Autodesk Inventor part; units mm, degrees
ref_plane "YZ Plane" through (0, 0, 0) normal (1, 0, 0) x (0, 1, 0)
ref_plane "XZ Plane" through (0, 0, 0) normal (0, 1, 0) x (-1, 0, 0)
ref_plane "XY Plane" through (0, 0, 0) normal (0, 0, 1) x (1, 0, 0)
sketch "Boceto1" plane through (0, 0, 0) normal (0, 1, 0) x (-1, 0, 0)
  line L0 (-71.0974, 28.13) -> (-71.0974, -25.87)
  line L1 (-71.0974, -25.87) -> (27.9026, -25.87)
  line L2 (27.9026, -25.87) -> (27.9026, 28.13)
  line L3 (4.4026, 48.13) -> (-47.5974, 48.13)
  line L4 (-47.5974, 48.13) -> (-47.5974, 28.13)
  line L5 (4.4026, 28.13) -> (4.4026, 48.13)
  line L6 (27.9026, 28.13) -> (4.4026, 28.13)
  line L7 (-47.5974, 28.13) -> (-71.0974, 28.13)
  circle A0 centre (-5.5974, 32.13) radius 2
  line L8 (-21.5974, 48.13) -> (-21.5974, -25.87)
  circle A1 centre (-37.5974, 32.13) radius 2
  line L9 (22.9026, -12.37) -> (6.9026, -12.37)
  line L10 (6.9026, -12.37) -> (6.9026, -23.37)
  line L11 (6.9026, -23.37) -> (22.9026, -23.37)
  line L12 (22.9026, -23.37) -> (22.9026, -12.37)
  line L13 (-66.0974, -12.37) -> (-50.0974, -12.37)
  line L14 (-50.0974, -12.37) -> (-50.0974, -23.37)
  line L15 (-50.0974, -23.37) -> (-66.0974, -23.37)
  line L16 (-66.0974, -23.37) -> (-66.0974, -12.37)
  circle A2 centre (-8.0974, -16.37) radius 2
  circle A3 centre (-35.0974, -16.37) radius 2
  point P0 (0, 0)
  dimension "d0" = 54
  dimension "d1" = 99
  dimension "d2" = 20
  dimension "d3" = 52
  dimension "d4" = 23.5
  dimension "d5" = 23.5
  dimension "d6" = 4
  dimension "d7" = 16
  dimension "d8" = 10
  dimension "d9" = 2.5
  dimension "d10" = 5
  dimension "d11" = 11
  dimension "d12" = 16
  dimension "d13" = 4
  dimension "d15" = 9.5
  dimension "d18" = 34
  dimension "d19" = 15
extrude "Extrusión1" add sketch "Boceto1" along normal blind 3.4
equation "\"Radio_pliegue\" = Grosor"
equation "\"Anchura_desahogo_plegado\" = Grosor"
equation "\"Profundidad_desahogo_plegado\" = 0.5 * Grosor"
equation "\"Tamaño_destalonado\" = 4 * Grosor"
equation "\"Remanente_mínimo\" = 2 * Grosor"
equation "\"Radiodetransición\" = Radio_pliegue"
equation "\"Tamaño_de_radio_de_Jacobi\" = Radio_pliegue"
equation "\"TamañoSeparación\" = Grosor"
properties part number "PlacaInferior"
Work out the finished part from the listing and answer in its coordinate system (mm). A direction names the side the tool comes from. Give positions to 0.01 mm unless a question says otherwise; leave off trailing zeros. Loops run counter-clockwise (first coordinate to the right, second up) from the corner with the lowest first, then second, coordinate; pieces in that order, holes last. Notation, with made-up numbers: (17, 32) - (61, 32) arc R11 ccw to (61, 38) - close; hole circle Ø5 at (82, 14). An arc over 180 degrees is marked (long way). Answer in a Markdown table with one row per item. Add a question column.
Q1. A tool of negligible diameter and unlimited length cuts with its end or side. For faces 5 (the flat face through (59, 2, 28.13)), 6 (the flat face through (-16, 2, 28.13)), 7 (the flat face through (22, 2, -25.87)), 8 (the flat face through (-27.903, 2, 1)), 9 (the flat face through (58, 2, -12.37)), from which of +Z, -Z, +X, -X, +Y, -Y can it reach the whole face along a straight path? Write none if from no direction.
Q2. Determine the mould class of faces 1 (the cylindrical face through (37.095, 1.676, -16.458)), 2 (the flat face through (58, 2, -23.37)), 3 (the flat face through (47.597, 2, 38)), 4 (the flat face through (22, 3.4, 12)) for opening direction X: released by +X, released by -X, zero draft, split by the parting line, or undercut.
Q3. The part is cut by section A-A (z = -16.37). Determine the outline of the cut face in (x, y).
Q4. The part is cut by section C-C (z = 32.13). Determine the outline of the cut face in (x, y), and give its area (3 significant figures).
Q5. Each of these flat-tipped pins is pushed along its axis until it touches: P1, Ø1.7, axis at x = 63, y = 2, coming from the +Z side; P2, Ø1, axis at y = 2.5, z = 38.5, coming from the +X side; P3, Ø6, axis at x = 14, z = 36, coming from the -Y side. Where does it stop, or does it pass through?
Q6. The part is cut by section B-B (y = 2.8). Determine the outline of the cut face in (x, z), and give its area (3 significant figures).
Q7. Consider line 1 along X through (y, z) = (1.5, -19); line 2 along Z through (x, y) = (-13, 1.5); line 3 along X through (y, z) = (1.85, 30.5). Determine where each line is inside the solid, lowest interval first.
Q8. The part is cut by section D-D (z = 43.5). Determine the outline of the cut face in (x, y), and give its area (3 significant figures).
Solution:
| question | item | result |
|---|---|---|
| 1 | face 5 | +Z, +X, +Y, -Y |
| 1 | face 6 | +Z, -X, +Y, -Y |
| 1 | face 7 | -Z, +X, -X, +Y, -Y |
| 1 | face 8 | +Z, -Z, -X, +Y, -Y |
| 1 | face 9 | +Y, -Y |
| 2 | face 1 | undercut |
| 2 | face 2 | undercut |
| 2 | face 3 | released by +X |
| 2 | face 4 | zero draft |
| 3 | outline | (-27.9, 0) - (-22.9, 0) - (-22.9, 3.4) - (-27.9, 3.4) - close; (-6.9, 0) - (6.1, 0) - (6.1, 3.4) - (-6.9, 3.4) - close; (10.1, 0) - (33.1, 0) - (33.1, 3.4) - (10.1, 3.4) - close; (37.1, 0) - (50.1, 0) - (50.1, 3.4) - (37.1, 3.4) - close; (66.1, 0) - (71.1, 0) - (71.1, 3.4) - (66.1, 3.4) - close |
| 4 | outline | (-4.4, 0) - (3.6, 0) - (3.6, 3.4) - (-4.4, 3.4) - close; (7.6, 0) - (35.6, 0) - (35.6, 3.4) - (7.6, 3.4) - close; (39.6, 0) - (47.6, 0) - (47.6, 3.4) - (39.6, 3.4) - close |
| 4 | area | 150 mm² |
| 5 | P1 | stops at z = 28.13 |
| 5 | P2 | stops at x = 47.6 |
| 5 | P3 | stops at y = 0 |
| 6 | outline | (-27.9, -25.87) - (71.1, -25.87) - (71.1, 28.13) - (47.6, 28.13) - (47.6, 48.13) - (-4.4, 48.13) - (-4.4, 28.13) - (-27.9, 28.13) - close; hole (-22.9, -23.37) - (-6.9, -23.37) - (-6.9, -12.37) - (-22.9, -12.37) - close; hole circle Ø4 at (5.6, 32.13); hole circle Ø4 at (8.1, -16.37); hole circle Ø4 at (35.1, -16.37); hole circle Ø4 at (37.6, 32.13); hole (50.1, -23.37) - (66.1, -23.37) - (66.1, -12.37) - (50.1, -12.37) - close |
| 6 | area | 5,980 mm² |
| 7 | line 1 | x = -27.9 to -22.9, -6.9 to 50.1, 66.1 to 71.1 |
| 7 | line 2 | z = -25.87 to -23.37, -12.37 to 28.13 |
| 7 | line 3 | x = -4.4 to 4.44, 6.76 to 36.44, 38.76 to 47.6 |
| 8 | outline | (-4.4, 0) - (47.6, 0) - (47.6, 3.4) - (-4.4, 3.4) - close |
| 8 | area | 177 mm² |
